Geometry: see drawing. Coordinates: mm, zero at the bounding-box minimum. A direction names the side the tool comes from. Round coordinates to 2 decimals unless told otherwise and drop trailing zeros. Loops run counter-clockwise (first coordinate to the right, second up) from the corner with the lowest first, then second, coordinate; pieces in that order, holes last. Notation, with made-up numbers: M 80.5,63.25 L 131.5,63.25 A13 cw 131.5,76.25 Z; hole C 3,81 d11. An arc over 180 degrees is marked long. Answer as a JSON object with one key per item and string values.
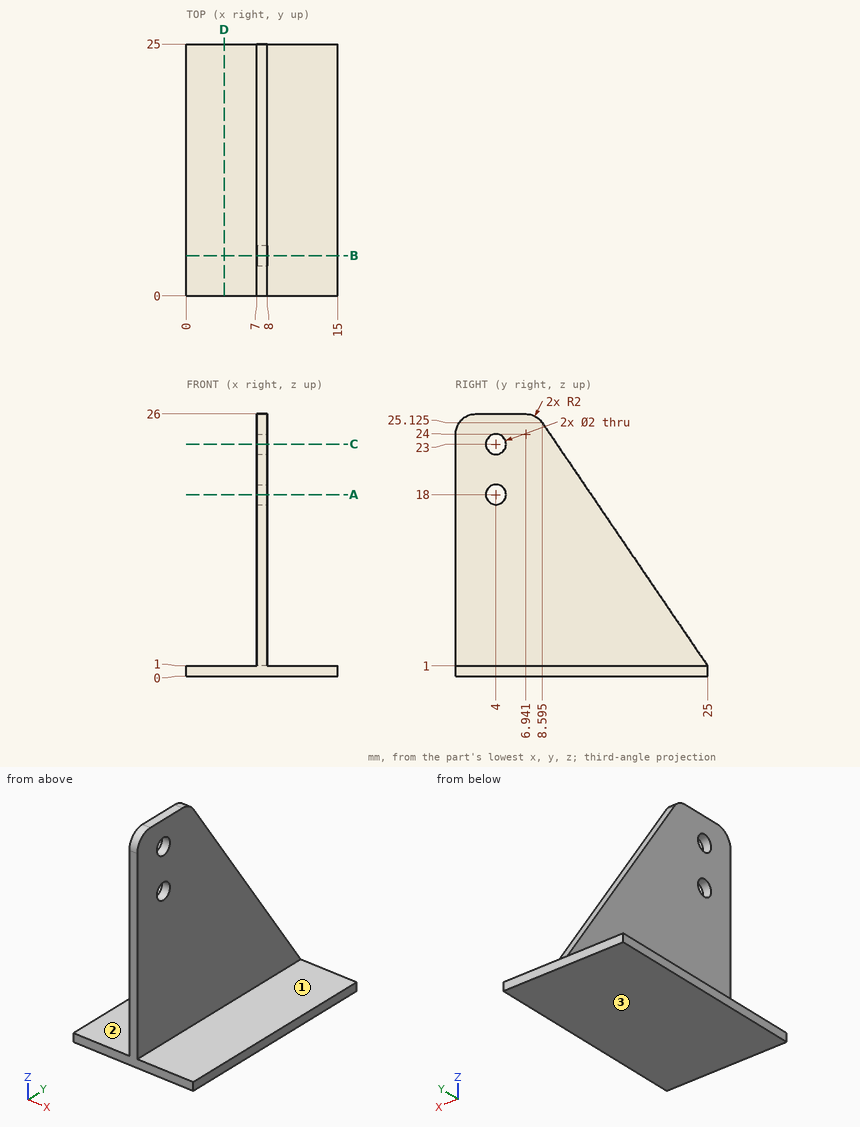
1) Section query A-A (z = 18). Return the cut outline in (x, y).
Results:
{"outline": "M 7,0 L 8,0 L 8,3 L 7,3 Z; M 7,5 L 8,5 L 8,13.44 L 7,13.44 Z"}
2) Section query D-D (x = 3.75). Return the cut outline in (y, z), and give its area (3 significant figures).
Results:
{"outline": "M 0,0 L 25,0 L 25,1 L 0,1 Z", "area": "25.0 mm2"}
3) Ray query, line 1 (Z direction, x = 7.6, y = 4); line 2 (Z direction, x = 3.25, y = 12); line 3 (X direction, y = 8.75, z = 11.5). Return the intervals inside material, ascending.
Results:
{"line 1": "0 to 17, 19 to 22, 24 to 26", "line 2": "0 to 1", "line 3": "7 to 8"}
4) Section query B-B (y = 4). Return the cut outline in (x, z).
Results:
{"outline": "M 0,0 L 15,0 L 15,1 L 8,1 L 8,17 L 7,17 L 7,1 L 0,1 Z; M 7,19 L 8,19 L 8,22 L 7,22 Z; M 7,24 L 8,24 L 8,26 L 7,26 Z"}
5) Section query C-C (z = 23). Return the cut outline in (x, y).
Results:
{"outline": "M 7,0 L 8,0 L 8,3 L 7,3 Z; M 7,5 L 8,5 L 8,10.04 L 7,10.04 Z"}
6) Reachability of the marked faces 1, 2 and 3 from +Z, -Z, +X, -X, +Y, -Y: full face, straight path, thin tool, end or side. Return the list, or none.
Results:
{"face 1": "+Z, +X, +Y, -Y", "face 2": "+Z, -X, +Y, -Y", "face 3": "-Z, +X, -X, +Y, -Y"}
7) Pin query (flat end, axial travel): P1, Ø10, axis at y = 17, z = 7.5, coming from the -X side; P2, Ø5.5, axis at x = 2.5, y = 9, coming from the +Z side; P3, Ø2, axis at x = 7.5, y = 2.5, coming from the -Z side; P4, Ø6, axis at y = 10.5, z = 17, coming from the +X side. Return the tip coordinate at first contact, or that it passes through.
Results:
{"P1": "x = 7", "P2": "z = 1", "P3": "z = 0", "P4": "x = 8"}
